from build123d import *

# Parameters (mm, degrees)
F0_R     = 38.1
F0_R_2   = 6.35
F1_DEPTH = 25.4
F2_R     = 5.08


with BuildPart() as f1:
    # F0 (on Top) → F1 (new body)
    with BuildSketch(Plane.XY):
        Circle(F0_R)
        with BuildLine():
            Line((-31.10852, -6.35), (-6.35, -6.35))
            Line((-6.35, -6.35), (-6.35, -31.10852))
            ThreePointArc((-6.35, -31.10852), (-22.45064, -22.45064), (-31.10852, -6.35))
        make_face(mode=Mode.SUBTRACT)
        with BuildLine():
            Line((6.35, -31.10852), (6.35, -6.35))
            Line((6.35, -6.35), (31.10852, -6.35))
            ThreePointArc((31.10852, -6.35), (22.45064, -22.45064), (6.35, -31.10852))
        make_face(mode=Mode.SUBTRACT)
        with BuildLine():
            Line((-6.35, 31.10852), (-6.35, 6.35))
            Line((-6.35, 6.35), (-31.10852, 6.35))
            ThreePointArc((-31.10852, 6.35), (-22.45064, 22.45064), (-6.35, 31.10852))
        make_face(mode=Mode.SUBTRACT)
        Circle(F0_R_2, mode=Mode.SUBTRACT)
        with BuildLine():
            ThreePointArc((6.35, 31.10852), (22.45064, 22.45064), (31.10852, 6.35))
            Line((31.10852, 6.35), (6.35, 6.35))
            Line((6.35, 6.35), (6.35, 31.10852))
        make_face(mode=Mode.SUBTRACT)
    extrude(amount=F1_DEPTH)

    # F2
    f2_edges = [f1.edges().sort_by_distance(p)[0] for p in [
        (38.1, 0, 12.7),
        (-38.1, 0, 0),
        (-38.1, 0, 25.4),
    ]]
    fillet(f2_edges, radius=F2_R)


solid = f1.part
Input: part model. Units: mm. Frame: model coordinates. A direction names the side the tool comes from. Coordinates: 2 decimals unless noted, no trailing zeros. Order: outer loops, then holes, each group sorted by start corner. A loop starts at its lowest first (then second) coordinate and runs counter-clockwise, first axis right, second up. Notation, with made-up numbers: M 57,71.5 L 78,71.5 A20 ccw 78,109.5 Z; hole C 67,-8 d4. An arc over 180 degrees is marked long. Answer in a Markdown table with one row per item.
(1) Section query D-D, the plane y = -15. Give the number of separate pieces and of enclosed holes in the cut face, plus the area to 3 significant figures.
Numbers:
| item | result |
|---|---|
| separate pieces | 3 |
| enclosed holes | 0 |
| area | 656 mm^2 |
(2) Material intervals for line 1 (Y direction, x = 15.5, z = 7.25); line 2 (Y direction, x = 0, z = 12.75); line 3 (Y direction, x = 13, z = 11), sorted ascending. Write a range as [from, to].
Numbers:
| item | result |
|---|---|
| line 1 | y = [-34.8, -27.71], [-6.35, 6.35], [27.71, 34.8] |
| line 2 | y = [-38.1, -6.35], [6.35, 38.1] |
| line 3 | y = [-35.81, -28.97], [-6.35, 6.35], [28.97, 35.81] |
(3) Access query for faces 4 (the flat face through (-5, 5, 0)), 5 (the flat face through (19, -6.35, 13)). Directions: +Z, -Z, +X, -X, +Y, -Y. A direction counts if a zero-diameter tool reaches every point of the face in a straight line with its end or side. Return the directions, or none.
Numbers:
| item | result |
|---|---|
| face 4 | -Z, +X, -X, +Y, -Y |
| face 5 | +Z, -Z |
(4) Section query B-B, the plane z = 8.5. Output: boundary loops of the cut face in (x, y).
Numbers:
| item | result |
|---|---|
| outline | C 0,0 d76.2; hole M -31.11,-6.35 A31.75 ccw -6.35,-31.11 L -6.35,-6.35 Z; hole M -31.11,6.35 L -6.35,6.35 L -6.35,31.11 A31.75 ccw Z; hole C 0,0 d12.7; hole M 6.35,-31.11 A31.75 ccw 31.11,-6.35 L 6.35,-6.35 Z; hole M 6.35,6.35 L 31.11,6.35 A31.75 ccw 6.35,31.11 Z |
(5) Draft query along X for faces 1 (the cylindrical face through (-30.235, -23.183, 12.593)), 2 (the flat face through (-19, -6.35, 13)), 3 (the flat face through (-5, 5, 25.4)). Return one class per face: pulls with the +X half, pulls with the -X half, needs draft (parallel to the pull), parting line crosses it, or undercut.
Numbers:
| item | result |
|---|---|
| face 1 | parting line crosses it |
| face 2 | undercut |
| face 3 | needs draft |
(6) Contact query for flat-ended pins moving along their axis: pin 1 Ø1 at (x, z) = (-30, 15.5) entering from -Y; pin 2 Ø5 at (y, z) = (-21.5, 8.5) entering from +X; pin 3 Ø5 at (x, y) = (-10, 5) entering from -Z; pin 4 Ø12 at (y, z) = (14, 22.5) entering from -X. Output: stop coordinate, or through.
Numbers:
| item | result |
|---|---|
| pin 1 | stops at y = -24.11 |
| pin 2 | stops at x = 33.02 |
| pin 3 | stops at z = 0 |
| pin 4 | stops at x = -37.18 |
(7) Section query A-A, the plane y = 0. Output: boundary loops of the cut face in (x, z).
Numbers:
| item | result |
|---|---|
| outline | M -38.1,5.08 A5.08 ccw -33.02,0 L -6.35,0 L -6.35,25.4 L -33.02,25.4 A5.08 ccw -38.1,20.32 Z; M 6.35,0 L 33.02,0 A5.08 ccw 38.1,5.08 L 38.1,20.32 A5.08 ccw 33.02,25.4 L 6.35,25.4 Z |
